```python
from build123d import *

# Parameters (mm, degrees)
CROQUIS1_W              = 148
CROQUIS1_H              = 25
SALIENTE_EXTRUIR1_DEPTH = 11
REDONDEO1_R             = 5
CROQUIS2_R              = 5.875
CORTAR_EXTRUIR1_DEPTH   = 9
CROQUIS3_R              = 7
CORTAR_EXTRUIR2_DEPTH   = 4.5


with BuildPart() as part:
    # Croquis1 → Saliente-Extruir1 (new body)
    with BuildSketch(Plane.XY):
        with Locations((38.75, -35)):
            Rectangle(CROQUIS1_W, CROQUIS1_H)
    extrude(amount=SALIENTE_EXTRUIR1_DEPTH)

    # Redondeo1
    redondeo1_edges = [part.edges().sort_by_distance(p)[0] for p in [
        (112.75, -35, 11),
        (38.75, -22.5, 11),
        (-35.25, -35, 11),
        (38.75, -47.5, 11),
    ]]
    fillet(redondeo1_edges, radius=REDONDEO1_R)

    # Croquis2 → Cortar-Extruir1 (cut)
    with BuildSketch(Plane(origin=(0, 0, 0), x_dir=(-1, 0, 0), z_dir=(0, 0, -1))):
        with Locations((-73.75, -35)):
            Circle(CROQUIS2_R)
        with Locations(Location((-3.75, -35, 0), (0, 0, 180))):  # turned: the seam where the file's is
            Circle(CROQUIS2_R)
    extrude(amount=-CORTAR_EXTRUIR1_DEPTH, mode=Mode.SUBTRACT)

    # Croquis3 → Cortar-Extruir2 (cut)
    with BuildSketch(Plane(origin=(0, 0, 0), x_dir=(-1, 0, 0), z_dir=(0, 0, -1))):
        with Locations((-73.75, -35)):
            Circle(CROQUIS3_R)
        with Locations(Location((-3.75, -35, 0), (0, 0, 180))):  # turned: the seam where the file's is
            Circle(CROQUIS3_R)
    extrude(amount=-CORTAR_EXTRUIR2_DEPTH, mode=Mode.SUBTRACT)


solid = part.part
```
Verification items for the finished model (mm, model axes). A direction names the side the tool comes from. Coordinates: 2 decimals unless noted, no trailing zeros. Order: outer loops, then holes, each group sorted by start corner. A loop starts at its lowest first (then second) coordinate and runs counter-clockwise, first axis right, second up. Notation, with made-up numbers: (84.25, -34.75) -> (117.25, -34.75) arc R14 ccw to (117.25, -13.75) -> close; hole circle Ø4 at (70, 23). An arc over 180 degrees is marked (long way). Put each result on its own line as item: value. Start each with the question number.
1) Cross-section at B-B (x = 3.75). Enter the section's corners in (y, z) (3 decimals).
2) Go/stop test with flat-tipped pins: pin 1 (1.5 mm diameter, centred on x = 27, y = -26, fed in from +Z); pin 2 (1 mm diameter, centred on y = -27.5, z = 7.5, fed in from +X); pin 3 (3.5 mm diameter, centred on x = 73, y = -35.5, fed in from -Z); pin 4 (6 mm diameter, centred on x = -20, z = 8, fed in from -Y). Record where each tip stops, or that it passes through.
3) Cross-section at A-A (y = -35). Enter the section's corners in (x, z) (3 decimals).
4) Material ranges on L1, parallel to X at y = -35.5, z = 0.5; L2, parallel to Y at x = 73.75, z = 5.7 (3 decimals); L3, parallel to X at y = -38, z = 4, recorded low to high.
5) Release check for a two-part mould opening along Y. For faces 1 (the flat face through (75, -29, 4.5)), 2 (the cylindrical face through (39.79, -23.93, 9.5)), 3 (the flat face through (38, -47.5, 3)) record: pulls with the +Y half, pulls with the -Y half, needs draft (parallel to the pull), parting line crosses it, or undercut.
6) Cross-section at C-C (z = 7.75). Enter the section's corners in (x, y) (3 decimals).
7) Cross-section at D-D (x = -13.5). Enter the section's corners in (y, z).
8) Tool access check on faces 4 (the flat face through (38, -35, 0)), 5 (the flat face through (74, -35, 9)). Record the directions out of +Z, -Z, +X, -X, +Y, -Y that give a thin tool (end or side, any length) a straight path to the whole face; none if there is none.
Geometry check:
1. outline: (-47.5, 0) -> (-42, 0) -> (-42, 4.5) -> (-40.875, 4.5) -> (-40.875, 9) -> (-29.125, 9) -> (-29.125, 4.5) -> (-28, 4.5) -> (-28, 0) -> (-22.5, 0) -> (-22.5, 6) arc R5 ccw to (-27.5, 11) -> (-42.5, 11) arc R5 ccw to (-47.5, 6) -> close
2. pin 1: stops at z = 10.94
2. pin 2: stops at x = 112.65
2. pin 3: stops at z = 9
2. pin 4: stops at y = -47.5
3. outline: (-35.25, 0) -> (-3.25, 0) -> (-3.25, 4.5) -> (-2.125, 4.5) -> (-2.125, 9) -> (9.625, 9) -> (9.625, 4.5) -> (10.75, 4.5) -> (10.75, 0) -> (66.75, 0) -> (66.75, 4.5) -> (67.875, 4.5) -> (67.875, 9) -> (79.625, 9) -> (79.625, 4.5) -> (80.75, 4.5) -> (80.75, 0) -> (112.75, 0) -> (112.75, 6) arc R5 ccw to (107.75, 11) -> (-30.25, 11) arc R5 ccw to (-35.25, 6) -> close
4. L1: x = -35.25 to -3.23, 10.73 to 66.77, 80.73 to 112.75
4. L2: y = -47.5 to -40.875, -29.125 to -22.5
4. L3: x = -35.25 to -2.57, 10.07 to 67.43, 80.07 to 112.75
5. face 1: undercut
5. face 2: pulls with the +Y half
5. face 3: pulls with the -Y half
6. outline: (-34.934, -47.184) -> (112.434, -47.184) -> (112.434, -22.816) -> (-34.934, -22.816) -> close; hole circle Ø11.75 at (3.75, -35); hole circle Ø11.75 at (73.75, -35)
7. outline: (-47.5, 0) -> (-22.5, 0) -> (-22.5, 6) arc R5 ccw to (-27.5, 11) -> (-42.5, 11) arc R5 ccw to (-47.5, 6) -> close
8. face 4: -Z, +X, -X, +Y, -Y
8. face 5: -Z
